from build123d import *

# Parameters (mm, degrees)
SKETCH1_W                               = 100
SKETCH1_H                               = 93.65
BOSS_EXTRUDE1_DEPTH                     = 6.35
TAP_DRILL_FOR_M3X0_5_TAP1_D             = 2.5
TAP_DRILL_FOR_M3X0_5_TAP1_DEPTH         = 9.248924226
TAP_DRILL_FOR_M3X0_5_TAP1_CSINK_D       = 2.55
TAP_DRILL_FOR_M3X0_5_TAP1_CSINK_ANGLE   = 90
TAP_DRILL_FOR_M3X0_5_TAP1_TIP           = 0.751075774
TAP_DRILL_FOR_M3X0_5_TAP2_D             = 2.5
TAP_DRILL_FOR_M3X0_5_TAP2_DEPTH         = 9.248924226
TAP_DRILL_FOR_M3X0_5_TAP2_CSINK_D       = 2.55
TAP_DRILL_FOR_M3X0_5_TAP2_CSINK_ANGLE   = 90
TAP_DRILL_FOR_M3X0_5_TAP2_TIP           = 0.751075774
TAP_DRILL_FOR_M12X1_75_TAP1_D           = 10.2
TAP_DRILL_FOR_M12X1_75_TAP1_CSINK_D     = 10.25
TAP_DRILL_FOR_M12X1_75_TAP1_CSINK_ANGLE = 90
SKETCH11_W                              = 5.7
SKETCH11_H                              = 2.6
CUT_EXTRUDE1_DEPTH                      = 69.796098182


with BuildPart() as part:
    # Sketch1 → Boss-Extrude1 (new body)
    with BuildSketch(Plane(origin=(0, 0, 0), x_dir=(1, 0, 0), z_dir=(0, 1, 0))):
        Rectangle(SKETCH1_W, SKETCH1_H)
    extrude(amount=BOSS_EXTRUDE1_DEPTH)

    # Tap Drill for M3x0.5 Tap1
    with Locations(Plane.XY.offset(46.825)):
        with Locations((-35, 3.175), (35, 3.175)):
            CounterSinkHole(TAP_DRILL_FOR_M3X0_5_TAP1_D / 2, TAP_DRILL_FOR_M3X0_5_TAP1_CSINK_D / 2, depth=TAP_DRILL_FOR_M3X0_5_TAP1_DEPTH, counter_sink_angle=TAP_DRILL_FOR_M3X0_5_TAP1_CSINK_ANGLE)
            with Locations((0, 0, -(TAP_DRILL_FOR_M3X0_5_TAP1_DEPTH + TAP_DRILL_FOR_M3X0_5_TAP1_TIP / 2))):  # 118° drill point
                Cone(0, TAP_DRILL_FOR_M3X0_5_TAP1_D / 2, TAP_DRILL_FOR_M3X0_5_TAP1_TIP, mode=Mode.SUBTRACT)

    # Tap Drill for M3x0.5 Tap2
    with Locations(Plane(origin=(0, 0, -46.825), x_dir=(-1, 0, 0), z_dir=(0, 0, -1))):
        with Locations((-35, 3.175), (35, 3.175)):
            CounterSinkHole(TAP_DRILL_FOR_M3X0_5_TAP2_D / 2, TAP_DRILL_FOR_M3X0_5_TAP2_CSINK_D / 2, depth=TAP_DRILL_FOR_M3X0_5_TAP2_DEPTH, counter_sink_angle=TAP_DRILL_FOR_M3X0_5_TAP2_CSINK_ANGLE)
            with Locations((0, 0, -(TAP_DRILL_FOR_M3X0_5_TAP2_DEPTH + TAP_DRILL_FOR_M3X0_5_TAP2_TIP / 2))):  # 118° drill point
                Cone(0, TAP_DRILL_FOR_M3X0_5_TAP2_D / 2, TAP_DRILL_FOR_M3X0_5_TAP2_TIP, mode=Mode.SUBTRACT)

    # Tap Drill for M12x1.75 Tap1 (through all)
    with Locations(Plane(origin=(0, 6.35, 0), x_dir=(1, 0, 0), z_dir=(0, 1, 0))):
        with Locations((0, 0)):
            CounterSinkHole(TAP_DRILL_FOR_M12X1_75_TAP1_D / 2, TAP_DRILL_FOR_M12X1_75_TAP1_CSINK_D / 2, counter_sink_angle=TAP_DRILL_FOR_M12X1_75_TAP1_CSINK_ANGLE)

    # Sketch11 → Cut-Extrude1 (cut, through all)
    with BuildSketch(Plane(origin=(0, 6.35, 0), x_dir=(1, 0, 0), z_dir=(0, 1, 0))):
        with Locations((35, -43)):
            Rectangle(SKETCH11_W, SKETCH11_H)
        with Locations((-35, -43)):
            Rectangle(SKETCH11_W, SKETCH11_H)
        with Locations((-35, 43.025)):
            Rectangle(SKETCH11_W, SKETCH11_H)
        with Locations((35, 43.025)):
            Rectangle(SKETCH11_W, SKETCH11_H)
    extrude(amount=-CUT_EXTRUDE1_DEPTH, mode=Mode.SUBTRACT)


solid = part.part
Input: part model. Units: mm. Frame: model coordinates. A direction names the side the tool comes from. Coordinates: 2 decimals unless noted, no trailing zeros. Loops run counter-clockwise (first coordinate to the right, second up) from the corner with the lowest first, then second, coordinate; pieces in that order, holes last. Notation, with made-up numbers: (36, -37.75) -> (83, -37.75) arc R14 cw to (83, -19.75) -> close; hole circle Ø6 at (42, 79). An arc over 180 degrees is marked (long way). One line per item, written item: value.
(1) Cut plane A-A (z = 0). Output: boundary loops of the cut face in (x, y) (3 decimals).
Answer below:
outline: (-50, 0) -> (-5.1, 0) -> (-5.1, 6.325) -> (-5.125, 6.35) -> (-50, 6.35) -> close; (5.1, 0) -> (50, 0) -> (50, 6.35) -> (5.125, 6.35) -> (5.1, 6.325) -> close
(2) Cut plane B-B (x = 0). Output: boundary loops of the cut face in (y, z) (3 decimals).
Answer below:
outline: (0, -46.825) -> (6.35, -46.825) -> (6.35, -5.125) -> (6.325, -5.1) -> (0, -5.1) -> close; (0, 5.1) -> (6.325, 5.1) -> (6.35, 5.125) -> (6.35, 46.825) -> (0, 46.825) -> close
(3) Draft query along Y for faces 6 (the face through (35.207, 3.24, 36.955)), 7 (the face through (-35, 5, 41.7)). Return one class per face: pulls with the +Y half, pulls with the -Y half, needs draft (parallel to the pull), parting line crosses it, or undercut.
Answer below:
face 6: undercut
face 7: needs draft
(4) Pin query (flat end, axial travel): pin 1 Ø3 at (x, y) = (-35, 3.175) entering from -Z (3 decimals); pin 2 Ø2 at (x, y) = (35, 3.175) entering from -Z. Return the tip coordinate at first contact, or that it passes through.
Answer below:
pin 1: stops at z = -46.825
pin 2: stops at z = -37.43
(5) Set-up query: faces 1 (the face through (33.75, 3.23, -45.55)), 2 (the face through (-35, 5, -44.325)), 3 (the face through (-50, 3, 1)), 4 (the face through (-33.75, 3.23, 39.61)), 5 (the face through (-1, 3, -46.825)). Return all of +Z, -Z, +X, -X, +Y, -Y with unobstructed straight access to the full face (end or side cutting, diameter ignored); none if empty.
Answer below:
face 1: -Z
face 2: +Y, -Y
face 3: +Z, -Z, -X, +Y, -Y
face 4: +Z
face 5: -Z, +X, -X, +Y, -Y
(6) Ray query, line 1 along X through (y, z) = (3.5, 42); line 2 along Y through (x, z) = (-35, 39) (3 decimals); line 3 along Z through (x, y) = (-2, 1.5) (3 decimals). Return the intervals inside material, ascending.
Answer below:
line 1: x = -50 to -37.85, -32.15 to 32.15, 37.85 to 50
line 2: y = 0 to 1.925, 4.425 to 6.35
line 3: z = -46.825 to -4.691, 4.691 to 46.825
